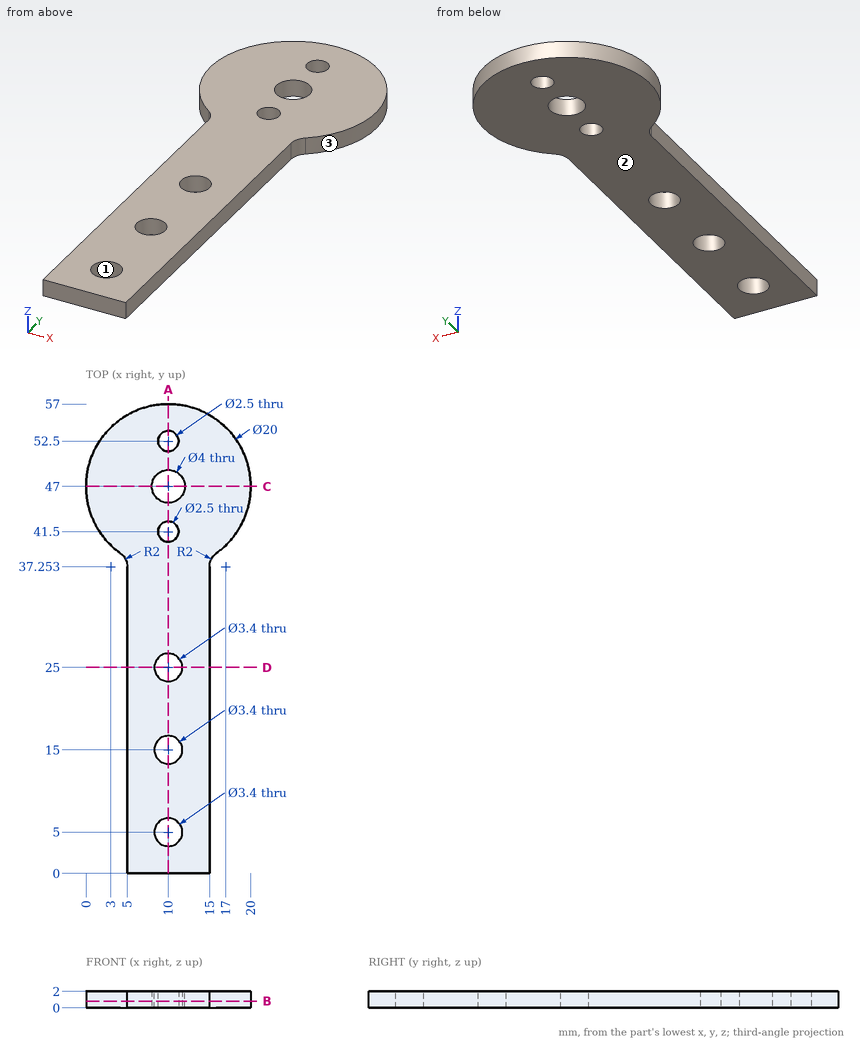
Can you work these out from the drawing? Everything is in mm from the part's minimum corner. Round coordinates to 2 decimals unless told otherwise and drop trailing zeros. Loops run counter-clockwise (first coordinate to the right, second up) from the corner with the lowest first, then second, coordinate; pieces in that order, holes last.
1. If we section it at D-D on y = 25: Write out the boundary of the cut face in (x, z), plus the area to 3 significant figures.
Answer list:
outline: (5, 0) - (8.3, 0) - (8.3, 2) - (5, 2) - close; (11.7, 0) - (15, 0) - (15, 2) - (11.7, 2) - close
area: 13.2 mm2
2. If we section it at A-A on x = 10: Write out the boundary of the cut face in (y, z).
Answer list:
outline: (0, 0) - (3.3, 0) - (3.3, 2) - (0, 2) - close; (6.7, 0) - (13.3, 0) - (13.3, 2) - (6.7, 2) - close; (16.7, 0) - (23.3, 0) - (23.3, 2) - (16.7, 2) - close; (26.7, 0) - (40.25, 0) - (40.25, 2) - (26.7, 2) - close; (42.75, 0) - (45, 0) - (45, 2) - (42.75, 2) - close; (49, 0) - (51.25, 0) - (51.25, 2) - (49, 2) - close; (53.75, 0) - (57, 0) - (57, 2) - (53.75, 2) - close
3. We'd pull the mould along Y, two halves only. Please class the marked faces 1, 2 and 3: +Y half, -Y half, draft (parallel to the pull), parting line (faces both ways), or undercut.
Answer list:
face 1: undercut
face 2: draft
face 3: parting line
4. If we section it at C-C on y = 47: Write out the boundary of the cut face in (x, z), plus the area to 3 significant figures.
Answer list:
outline: (0, 0) - (8, 0) - (8, 2) - (0, 2) - close; (12, 0) - (20, 0) - (20, 2) - (12, 2) - close
area: 32.0 mm2
5. For P1, Ø3, axis at x = 10, y = 52.5, coming from the -Z side; P2, Ø1, axis at y = 10.5, z = 1.5, coming from the +X side; P3, Ø0.6, axis at y = 9.5, z = 1, coming from the -X side, each with a flat end and sliding along its axis, tell me the tip position at first contact or that it passes through.
Answer list:
P1: stops at z = 0
P2: stops at x = 15
P3: stops at x = 5
6. If I drill on line 1 along X through (y, z) = (47, 1.2); line 2 along X through (y, z) = (48, 0.6); line 3 along X through (y, z) = (32, 0.8), over which ranges is the centre line in solid material (lowest first)?
Answer list:
line 1: x = 0 to 8, 12 to 20
line 2: x = 0.05 to 8.27, 11.73 to 19.95
line 3: x = 5 to 15
7. If we section it at B-B on z = 0.8: Write out the boundary of the cut face in (x, y).
Answer list:
outline: (4.17, 38.88) arc R2 cw to (5, 37.25) - (5, 0) - (15, 0) - (15, 37.25) arc R2 cw to (15.83, 38.88) arc R10 ccw (long way) to start; hole circle Ø4 at (10, 47); hole circle Ø3.4 at (10, 5); hole circle Ø3.4 at (10, 15); hole circle Ø3.4 at (10, 25); hole circle Ø2.5 at (10, 41.5); hole circle Ø2.5 at (10, 52.5)
